Source: three-view drawing plus pictorial views. Frame: mm from the lowest corner of the part. A direction names the side the tool comes from. Give positions to 0.01 mm unless a question says otherwise; leave off trailing zeros. Loops run counter-clockwise (first coordinate to the right, second up) from the corner with the lowest first, then second, coordinate; pieces in that order, holes last.
1. Material intervals for line 1 along Z through (x, y) = (10, 1.4); line 2 along X through (y, z) = (5.3, 3); line 3 along X through (y, z) = (2.9, 27), sorted ascending.
2. Draft query along X for the marked faces 6, 7, 8 and 9. Return one class per face: +X half, -X half, draft (parallel to the pull), parting line (faces both ways), or undercut.
3. Section D-D, the plane y = 6.25. Output: boundary loops of the cut face in (x, z), then the cut area to 3 significant figures.
4. First-contact query: P1, Ø7, axis at x = 17.5, z = 15.5, coming from the -Y side; P2, Ø0.5, axis at y = 0.5, z = 0.5, coming from the -X side; P3, Ø5, axis at x = 10, z = 27, coming from the +Y side; P4, Ø3, axis at x = 10, z = 15, coming from the +Y side. Flat tips, straight axial feed; report the tip coordinate or a pass-through.
5. Section C-C, the plane z = 15. Output: boundary loops of the cut face in (x, y), then the cut area to 3 significant figures.
6. Section B-B, the plane y = 3.5. Output: boundary loops of the cut face in (x, z).
7. Section A-A, the plane z = 3. Output: boundary loops of the cut face in (x, y).
8. Access query for the marked faces 1, 2, 3, 4 and 5. Directions: +Z, -Z, +X, -X, +Y, -Y. A direction counts if a zero-diameter tool reaches every point of the face in a straight line with its end or side. Return the directions, or none.
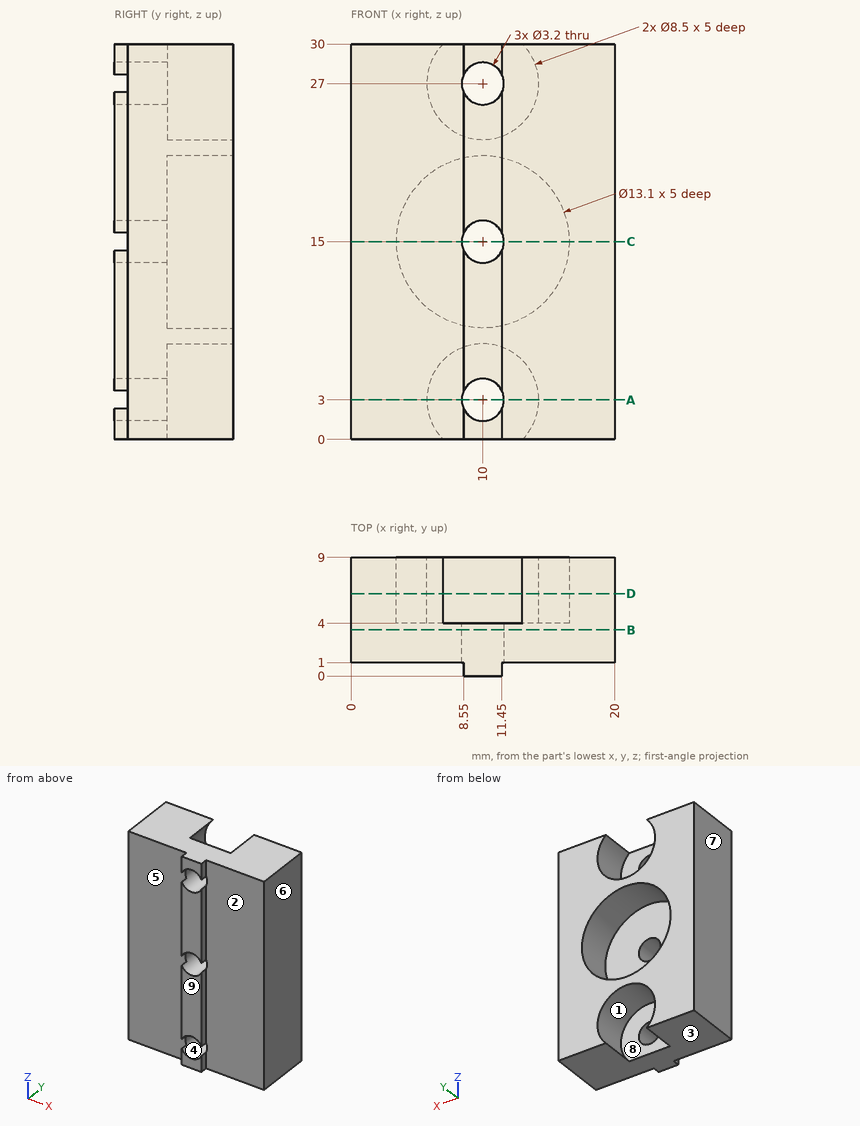
Answers below:
1. line 1: z = 0 to 1.4, 4.6 to 13.4, 16.6 to 25.4, 28.6 to 30
1. line 2: x = 0 to 5.75, 14.25 to 20
1. line 3: x = 0 to 8.4, 11.6 to 20
2. face 6: +X half
2. face 7: -X half
2. face 8: undercut
2. face 9: draft
3. outline: (0, 0) - (6.99, 0) arc R4.25 cw (long way) to (13.01, 0) - (20, 0) - (20, 30) - (13.01, 30) arc R4.25 cw (long way) to (6.99, 30) - (0, 30) - close; hole circle Ø13.1 at (10, 15)
3. area: 362 mm2
4. P1: stops at y = 1
4. P2: stops at x = 8.55
4. P3: stops at y = 4
4. P4: passes through
5. outline: (0, 1) - (8.4, 1) - (8.4, 4) - (3.45, 4) - (3.45, 9) - (0, 9) - close; (11.6, 1) - (20, 1) - (20, 9) - (16.55, 9) - (16.55, 4) - (11.6, 4) - close
5. area: 84.9 mm2
6. outline: (0, 0) - (20, 0) - (20, 30) - (0, 30) - close; hole circle Ø3.2 at (10, 3); hole circle Ø3.2 at (10, 15); hole circle Ø3.2 at (10, 27)
7. outline: (0, 1) - (8.4, 1) - (8.4, 4) - (5.75, 4) - (5.75, 9) - (0, 9) - close; (11.6, 1) - (20, 1) - (20, 9) - (14.25, 9) - (14.25, 4) - (11.6, 4) - close
8. face 1: +Y
8. face 2: +Z, -Z, +X, -Y
8. face 3: -Z, +X, -X, +Y, -Y
8. face 4: +Y, -Y
8. face 5: +Z, -Z, -X, -Y
